```python
from build123d import *

# Parameters (mm, degrees)
SKETCH1_W                = 107.95
SKETCH1_H                = 25.4
BOSS_EXTRUDE1_DEPTH      = 7.62
SKETCH2_W                = 2.032
SKETCH2_H                = 25.4
CUT_EXTRUDE1_DEPTH       = 1.143
LPATTERN1_COUNT          = 10
LPATTERN1_PITCH          = 3.175
MIRROR1_COPY_1_SKETCH_W  = 2.032
MIRROR1_COPY_1_SKETCH_H  = 25.4
MIRROR1_COPY_1_DEPTH     = 1.143
MIRROR1_COPY_2_SKETCH_W  = 2.032
MIRROR1_COPY_2_SKETCH_H  = 25.4
MIRROR1_COPY_2_DEPTH     = 1.143
MIRROR1_COPY_3_SKETCH_W  = 2.032
MIRROR1_COPY_3_SKETCH_H  = 25.4
MIRROR1_COPY_3_DEPTH     = 1.143
MIRROR1_COPY_4_SKETCH_W  = 2.032
MIRROR1_COPY_4_SKETCH_H  = 25.4
MIRROR1_COPY_4_DEPTH     = 1.143
MIRROR1_COPY_5_SKETCH_W  = 2.032
MIRROR1_COPY_5_SKETCH_H  = 25.4
MIRROR1_COPY_5_DEPTH     = 1.143
MIRROR1_COPY_6_SKETCH_W  = 2.032
MIRROR1_COPY_6_SKETCH_H  = 25.4
MIRROR1_COPY_6_DEPTH     = 1.143
MIRROR1_COPY_7_SKETCH_W  = 2.032
MIRROR1_COPY_7_SKETCH_H  = 25.4
MIRROR1_COPY_7_DEPTH     = 1.143
MIRROR1_COPY_8_SKETCH_W  = 2.032
MIRROR1_COPY_8_SKETCH_H  = 25.4
MIRROR1_COPY_8_DEPTH     = 1.143
MIRROR1_COPY_9_SKETCH_W  = 2.032
MIRROR1_COPY_9_SKETCH_H  = 25.4
MIRROR1_COPY_9_DEPTH     = 1.143
MIRROR1_COPY_10_SKETCH_W = 2.032
MIRROR1_COPY_10_SKETCH_H = 25.4
MIRROR1_COPY_10_DEPTH    = 1.143
SKETCH3_R                = 2.499995
CUT_EXTRUDE2_DEPTH       = 56.970126184


with BuildPart() as part:
    # Sketch1 → Boss-Extrude1 (new body)
    with BuildSketch(Plane(origin=(0, 0, 0), x_dir=(1, 0, 0), z_dir=(0, 1, 0))):
        Rectangle(SKETCH1_W, SKETCH1_H)
        with BuildLine():
            Line((-31.75, 4.7625), (31.75, 4.7625))
            ThreePointArc((31.75, 4.7625), (36.5125, 0), (31.75, -4.7625))
            Line((31.75, -4.7625), (-31.75, -4.7625))
            ThreePointArc((-31.75, -4.7625), (-36.5125, 0), (-31.75, 4.7625))
        make_face(mode=Mode.SUBTRACT)
    extrude(amount=BOSS_EXTRUDE1_DEPTH)

    # Sketch2 → Cut-Extrude1 (cut)
    with BuildSketch(Plane(origin=(0, 7.62, 0), x_dir=(1, 0, 0), z_dir=(0, 1, 0))):
        Rectangle(SKETCH2_W, SKETCH2_H)
    cut_extrude1 = extrude(amount=-CUT_EXTRUDE1_DEPTH, mode=Mode.SUBTRACT)

    # LPattern1: Cut-Extrude1 ×10
    with Locations(*[(i * LPATTERN1_PITCH, 0, 0) for i in range(1, LPATTERN1_COUNT)]):
        add(cut_extrude1, mode=Mode.SUBTRACT)

    # Mirror1 copy 1 sketch → Mirror1 copy 1 (cut)
    with BuildSketch(Plane(origin=(-3.175, 7.62, 0), x_dir=(-1, 0, 0), z_dir=(0, 1, 0))):
        Rectangle(MIRROR1_COPY_1_SKETCH_W, MIRROR1_COPY_1_SKETCH_H)
    extrude(amount=-MIRROR1_COPY_1_DEPTH, mode=Mode.SUBTRACT)

    # Mirror1 copy 2 sketch → Mirror1 copy 2 (cut)
    with BuildSketch(Plane(origin=(-6.35, 7.62, 0), x_dir=(-1, 0, 0), z_dir=(0, 1, 0))):
        Rectangle(MIRROR1_COPY_2_SKETCH_W, MIRROR1_COPY_2_SKETCH_H)
    extrude(amount=-MIRROR1_COPY_2_DEPTH, mode=Mode.SUBTRACT)

    # Mirror1 copy 3 sketch → Mirror1 copy 3 (cut)
    with BuildSketch(Plane(origin=(-9.525, 7.62, 0), x_dir=(-1, 0, 0), z_dir=(0, 1, 0))):
        Rectangle(MIRROR1_COPY_3_SKETCH_W, MIRROR1_COPY_3_SKETCH_H)
    extrude(amount=-MIRROR1_COPY_3_DEPTH, mode=Mode.SUBTRACT)

    # Mirror1 copy 4 sketch → Mirror1 copy 4 (cut)
    with BuildSketch(Plane(origin=(-12.7, 7.62, 0), x_dir=(-1, 0, 0), z_dir=(0, 1, 0))):
        Rectangle(MIRROR1_COPY_4_SKETCH_W, MIRROR1_COPY_4_SKETCH_H)
    extrude(amount=-MIRROR1_COPY_4_DEPTH, mode=Mode.SUBTRACT)

    # Mirror1 copy 5 sketch → Mirror1 copy 5 (cut)
    with BuildSketch(Plane(origin=(-15.875, 7.62, 0), x_dir=(-1, 0, 0), z_dir=(0, 1, 0))):
        Rectangle(MIRROR1_COPY_5_SKETCH_W, MIRROR1_COPY_5_SKETCH_H)
    extrude(amount=-MIRROR1_COPY_5_DEPTH, mode=Mode.SUBTRACT)

    # Mirror1 copy 6 sketch → Mirror1 copy 6 (cut)
    with BuildSketch(Plane(origin=(-19.05, 7.62, 0), x_dir=(-1, 0, 0), z_dir=(0, 1, 0))):
        Rectangle(MIRROR1_COPY_6_SKETCH_W, MIRROR1_COPY_6_SKETCH_H)
    extrude(amount=-MIRROR1_COPY_6_DEPTH, mode=Mode.SUBTRACT)

    # Mirror1 copy 7 sketch → Mirror1 copy 7 (cut)
    with BuildSketch(Plane(origin=(-22.225, 7.62, 0), x_dir=(-1, 0, 0), z_dir=(0, 1, 0))):
        Rectangle(MIRROR1_COPY_7_SKETCH_W, MIRROR1_COPY_7_SKETCH_H)
    extrude(amount=-MIRROR1_COPY_7_DEPTH, mode=Mode.SUBTRACT)

    # Mirror1 copy 8 sketch → Mirror1 copy 8 (cut)
    with BuildSketch(Plane(origin=(-25.4, 7.62, 0), x_dir=(-1, 0, 0), z_dir=(0, 1, 0))):
        Rectangle(MIRROR1_COPY_8_SKETCH_W, MIRROR1_COPY_8_SKETCH_H)
    extrude(amount=-MIRROR1_COPY_8_DEPTH, mode=Mode.SUBTRACT)

    # Mirror1 copy 9 sketch → Mirror1 copy 9 (cut)
    with BuildSketch(Plane(origin=(-28.575, 7.62, 0), x_dir=(-1, 0, 0), z_dir=(0, 1, 0))):
        Rectangle(MIRROR1_COPY_9_SKETCH_W, MIRROR1_COPY_9_SKETCH_H)
    extrude(amount=-MIRROR1_COPY_9_DEPTH, mode=Mode.SUBTRACT)

    # Mirror1 copy 10 sketch → Mirror1 copy 10 (cut)
    with BuildSketch(Plane(origin=(0, 7.62, 0), x_dir=(-1, 0, 0), z_dir=(0, 1, 0))):
        Rectangle(MIRROR1_COPY_10_SKETCH_W, MIRROR1_COPY_10_SKETCH_H)
    extrude(amount=-MIRROR1_COPY_10_DEPTH, mode=Mode.SUBTRACT)

    # Sketch3 → Cut-Extrude2 (cut, through all)
    with BuildSketch(Plane(origin=(0, 7.62, 0), x_dir=(1, 0, 0), z_dir=(0, 1, 0))):
        with Locations(Location((-47.625, 0, 0), (0, 0, 270))):
            Circle(SKETCH3_R)
        with Locations(Location((47.625, 0, 0), (0, 0, 270))):
            Circle(SKETCH3_R)
    extrude(amount=-CUT_EXTRUDE2_DEPTH, mode=Mode.SUBTRACT)


solid = part.part
```
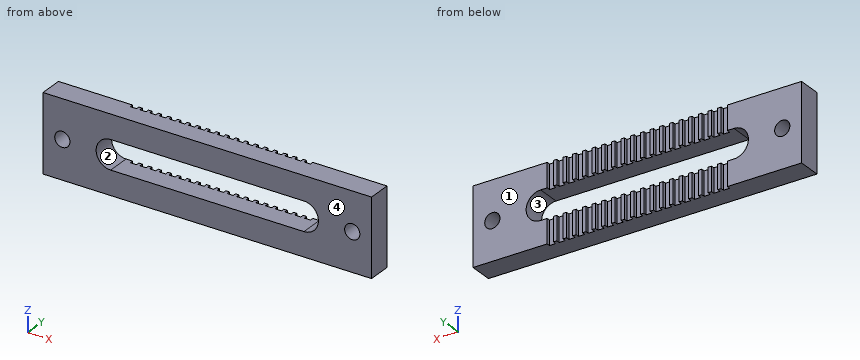
Model file for the job. Use its own axes, mm. Face numbers are marked on the shaded views. A direction names the side the tool comes from. Give positions to 0.01 mm unless a question says otherwise; leave off trailing zeros. Loops run counter-clockwise (first coordinate to the right, second up) from the corner with the lowest first, then second, coordinate; pieces in that order, holes last. Notation, with made-up numbers: (5, -11.5) -> (19, -11.5) arc R24 ccw to (19, 17.5) -> close; hole circle Ø2 at (75.25, 67). An arc over 180 degrees is marked (long way). Use CSV: the item, a comma, the result in double quotes. Start each with the question number.
1) Slice it at A-A on x = 0. Give the cut face in (y, z).
2) Flat gauge pin, fed straight in: pin 1 Ø1 at (x, z) = (-28.5, 7) entering from +Y. Where does the tip first touch, or does it go through?
3) Slice it at D-D on x = 35. Give the cut face in (y, z), plus the area to 3 significant figures.
4) Tool access for the marked faces 1 and 2: list every direction of +Z, -Z, +X, -X, +Y, -Y with a clear straight run to the whole face (end or side of a thin tool).
5) Slice it at B-B on z = 0. Give the cut face in (x, y) (1 decimal).
6) Mould opens along Z. For the marked faces 3 and 4 say: released by +Z, released by -Z, zero draft, split by the parting line, or undercut.
7) Slice it at C-C on y = 5.5. Give the number of separate pieces and of enclosed holes in the cut face, plus the area to 3 significant figures.
8) Wall check: line 1 (X direction, y = 3.25, z = 0) (1 decimal); line 2 (Z direction, x = 15, y = 2); line 3 (X direction, y = 5, z = -0.5) (3 decimals). Give the ranges that are in metal, low to high.
Computed values:
1,outline,"(0, -12.7) -> (6.48, -12.7) -> (6.48, -4.76) -> (0, -4.76) -> close; (0, 4.76) -> (6.48, 4.76) -> (6.48, 12.7) -> (0, 12.7) -> close"
2,pin 1,"stops at y = 6.48"
3,outline,"(0, -12.7) -> (7.62, -12.7) -> (7.62, -3.48) -> (0, -3.48) -> close; (0, 3.48) -> (7.62, 3.48) -> (7.62, 12.7) -> (0, 12.7) -> close"
3,area,"140 mm^2"
4,face 1,"+Z, -Z, +X, -X, +Y"
4,face 2,"+Y, -Y"
5,outline,"(-54, 0) -> (-50.1, 0) -> (-50.1, 7.6) -> (-54, 7.6) -> close; (-45.1, 0) -> (-36.5, 0) -> (-36.5, 7.6) -> (-45.1, 7.6) -> close; (36.5, 0) -> (45.1, 0) -> (45.1, 7.6) -> (36.5, 7.6) -> close; (50.1, 0) -> (54, 0) -> (54, 7.6) -> (50.1, 7.6) -> close"
6,face 3,"undercut"
6,face 4,"zero draft"
7,separate pieces,"1"
7,enclosed holes,"3"
7,area,"2,030 mm^2"
8,line 1,"x = -54 to -50.1, -45.1 to -36.5, 36.5 to 45.1, 50.1 to 54"
8,line 2,"z = -12.7 to -4.76, 4.76 to 12.7"
8,line 3,"x = -53.975 to -50.074, -45.176 to -36.486, 36.486 to 45.176, 50.074 to 53.975"
